The listing builds one solid part. Answer for the finished solid, in the listing's coordinates (mm). A direction names the side the tool comes from. Coordinates: 2 decimals unless noted, no trailing zeros. Order: outer loops, then holes, each group sorted by start corner. A loop starts at its lowest first (then second) coordinate and runs counter-clockwise, first axis right, second up. Notation, with made-up numbers: (67, 5) -> (115, 5) arc R21 cw to (115, 29) -> close; hole circle Ø3 at (33.25, -11). An arc over 180 degrees is marked (long way). Return JSON: item names as keys, results as strings.
```python
from build123d import *

# Parameters (mm, degrees)
SKETCH_21_W         = 15
SKETCH_21_H         = 15
SKETCH_21_W_2       = 13
SKETCH_21_H_2       = 13
F_15X15X1_1_DEPTH   = 488
SKETCH_3_R          = 1.5
CUT_EXTRUDE_1_DEPTH = 245.575652917


with BuildPart() as part:
    # 草图21 → 矩形管 方铝管15X15X1(1) (new body)
    with BuildSketch(Plane(origin=(-244, 0, 0), x_dir=(0, 0, -1), z_dir=(1, 0, 0))):
        Rectangle(SKETCH_21_W, SKETCH_21_H)
        Rectangle(SKETCH_21_W_2, SKETCH_21_H_2, mode=Mode.SUBTRACT)
    extrude(amount=F_15X15X1_1_DEPTH)

    # 草图3 → 切除-拉伸1 (cut, through all)
    with BuildSketch(Plane(origin=(0, -7.5, 0), x_dir=(1, 0, 0), z_dir=(0, 1, 0))):
        with Locations(Location((-224, 0, 0), (0, 0, 270))):
            Circle(SKETCH_3_R)
        with Locations(Location((-112, 0, 0), (0, 0, 270))):
            Circle(SKETCH_3_R)
        with Locations(Location((0, 0, 0), (0, 0, 270))):
            Circle(SKETCH_3_R)
        with Locations(Location((112, 0, 0), (0, 0, 270))):
            Circle(SKETCH_3_R)
        with Locations(Location((224, 0, 0), (0, 0, 270))):
            Circle(SKETCH_3_R)
    extrude(amount=CUT_EXTRUDE_1_DEPTH, mode=Mode.SUBTRACT)


solid = part.part
```
Item 1: Which of the six approach directions +Z, -Z, +X, -X, +Y, -Y give full straight-line access (tool end or side, diameter ignored) to faces 1 (the flat face through (-244, 0, 7)), 2 (the flat face through (-3, -6.5, 0))?
Answer list:
{"face 1": "+Z, -Z, -X, +Y, -Y", "face 2": "+X, -X"}
Item 2: Determine the mould class of faces 3 (the flat face through (-3, 6.5, 0)), 4 (the flat face through (-3, -7.5, 0)), 5 (the flat face through (-3, 0, -7.5)), 6 (the flat face through (-3, 7.5, 0)) for opening direction Y: pulls with the +Y half, pulls with the -Y half, needs draft (parallel to the pull), parting line crosses it, or undercut.
Answer list:
{"face 3": "undercut", "face 4": "pulls with the -Y half", "face 5": "needs draft", "face 6": "pulls with the +Y half"}
Item 3: The part is cut by section A-A on z = 4.25. Determine the outline of the cut face in (x, y).
Answer list:
{"outline": "(-244, -7.5) -> (244, -7.5) -> (244, -6.5) -> (-244, -6.5) -> close; (-244, 6.5) -> (244, 6.5) -> (244, 7.5) -> (-244, 7.5) -> close"}
Item 4: A flat-ended cylindrical pin translates along its axis: pin 1 (5 mm diameter, centred on x = 112, z = 0, fed in from +Y). Find the tip coordinate at first contact, or state that the pin passes through.
Answer list:
{"pin 1": "y = 7.5"}
Item 5: Find the intervals of material crossed by probe 1 along X at (y, z) = (7.2, 0); probe 2 along Z at (x, y) = (224, 6.8); probe 3 along Z at (x, y) = (-7, -4.75), in increasing order.
Answer list:
{"probe 1": "-244 to -225.5, -222.5 to -113.5, -110.5 to -1.5, 1.5 to 110.5, 113.5 to 222.5, 225.5 to 244", "probe 2": "-7.5 to -1.5, 1.5 to 7.5", "probe 3": "-7.5 to -6.5, 6.5 to 7.5"}
Item 6: The part is cut by section C-C on x = 190. Determine the outline of the cut face in (y, z).
Answer list:
{"outline": "(-7.5, -7.5) -> (7.5, -7.5) -> (7.5, 7.5) -> (-7.5, 7.5) -> close; hole (-6.5, -6.5) -> (6.5, -6.5) -> (6.5, 6.5) -> (-6.5, 6.5) -> close"}
